Verification items for the finished model (mm, model axes). A direction names the side the tool comes from. Round coordinates to 2 decimals unless told otherwise and drop trailing zeros. Write each loop counter-clockwise with the first axis right and the second up, starting at its lowest first coordinate (ties: lowest second). Pieces come first, ordered by that corner, then holes. Notation, with made-up numbers: M -15,-5.75 L 0,-5.75 A15 ccw 0,15.25 Z; hole C -33.75,80.5 d11. An arc over 180 degrees is marked long. Write each question's results on one line, items separated by ' | '.
from build123d import *

# Parameters (mm, degrees)
SKETCH1_W           = 20
SKETCH1_H           = 6
BOSS_EXTRUDE1_DEPTH = 6


with BuildPart() as part:
    # Sketch1 → Boss-Extrude1 (new body)
    with BuildSketch(Plane(origin=(0, 0, 0), x_dir=(1, 0, 0), z_dir=(0, 1, 0))):
        with BuildLine():
            Line((-10, 33), (10, 33))
            ThreePointArc((10, 33), (13.535533906, 31.535533906), (15, 28))
            Line((15, 28), (15, -2))
            ThreePointArc((15, -2), (13.535533906, -5.535533906), (10, -7))
            Line((10, -7), (-10, -7))
            ThreePointArc((-10, -7), (-13.535533906, -5.535533906), (-15, -2))
            Line((-15, -2), (-15, 28))
            ThreePointArc((-15, 28), (-13.535533906, 31.535533906), (-10, 33))
        make_face()
        with Locations((0, 26)):
            Rectangle(SKETCH1_W, SKETCH1_H, mode=Mode.SUBTRACT)
        Rectangle(SKETCH1_W, SKETCH1_H, mode=Mode.SUBTRACT)
    extrude(amount=BOSS_EXTRUDE1_DEPTH)


solid = part.part
1) Sectioned sample at D-D, the plane x = -13. Record the cut outline in (y, z), and give its area (3 significant figures).
Calculated:
outline: M 0,-32 L 6,-32 L 6,6 L 0,6 Z | area: 228 mm²
2) Access from +Z, -Z, +X, -X, +Y, -Y to the whole of each face (thin tool, end or side, straight path). Record for faces 4 (the flat face through (10, 3, 0)), 5 (the flat face through (0, 3, -33)).
Calculated:
face 4: +Y, -Y | face 5: -Z, +X, -X, +Y, -Y
3) Material ranges on line 1 (Z direction, x = 5.5, y = 0.5); line 2 (X direction, y = 5, z = -1.5); line 3 (Z direction, x = -10.25, y = 4.25), recorded low to high. Write a range as [from, to].
Calculated:
line 1: z = [-33, -29], [-23, -3], [3, 7] | line 2: x = [-15, -10], [10, 15] | line 3: z = [-32.99, 6.99]
4) Sectioned sample at B-B, the plane z = -26.5. Record the cut outline in (x, y).
Calculated:
outline: M -15,0 L -10,0 L -10,6 L -15,6 Z; M 10,0 L 15,0 L 15,6 L 10,6 Z
5) Sectioned sample at A-A, the plane x = -8. Record the cut outline in (y, z), and give its area (3 significant figures).
Calculated:
outline: M 0,-33 L 6,-33 L 6,-29 L 0,-29 Z; M 0,-23 L 6,-23 L 6,-3 L 0,-3 Z; M 0,3 L 6,3 L 6,7 L 0,7 Z | area: 168 mm²
6) Draft check along Z on faces 1 (the flat face through (-15, 3, -13)), 2 (the flat face through (0, 3, -23)), 3 (the cylindrical face through (-13, 3, 6)). Enter one of: pulls with the +Z half, pulls with the -Z half, needs draft (parallel to the pull), parting line crosses it, or undercut.
Calculated:
face 1: needs draft | face 2: undercut | face 3: pulls with the +Z half
7) Sectioned sample at C-C, the plane y = 3.2. Record the cut outline in (x, z), and give its area (3 significant figures).
Calculated:
outline: M -15,-28 A5 ccw -10,-33 L 10,-33 A5 ccw 15,-28 L 15,2 A5 ccw 10,7 L -10,7 A5 ccw -15,2 Z; hole M -10,-29 L 10,-29 L 10,-23 L -10,-23 Z; hole M -10,-3 L 10,-3 L 10,3 L -10,3 Z | area: 939 mm²
